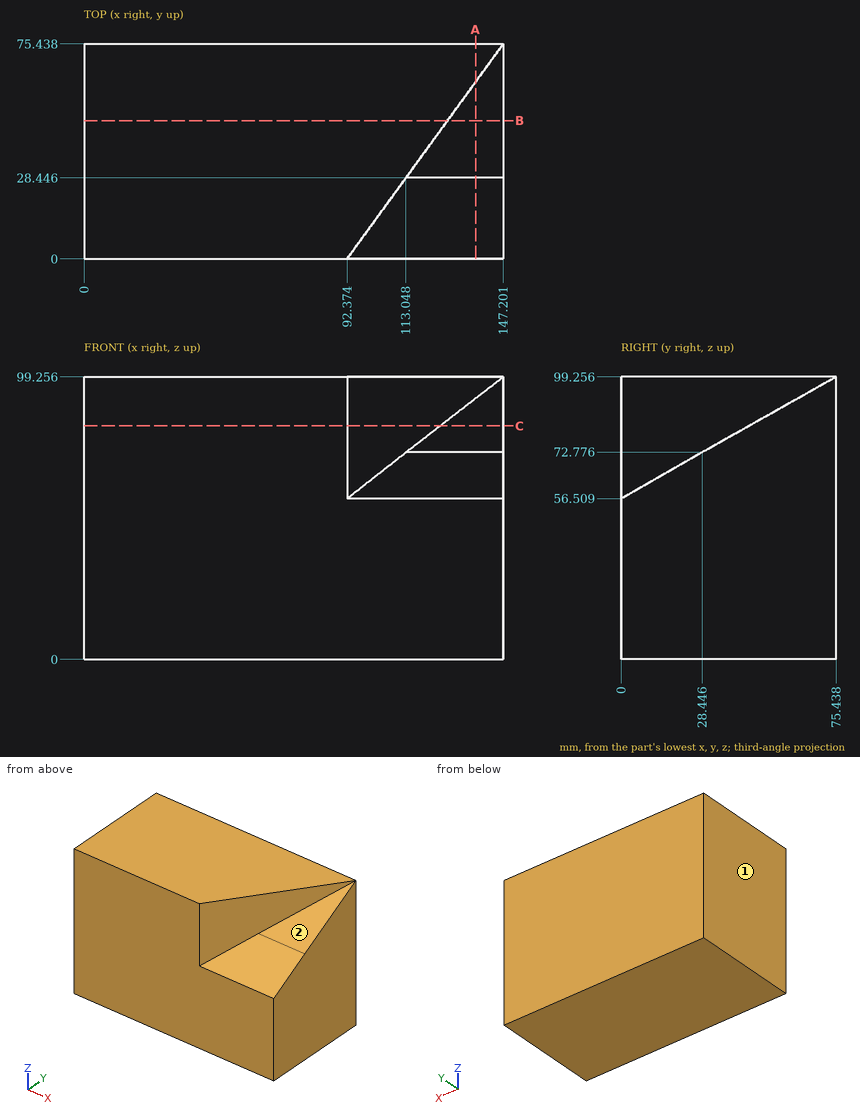
Source: three-view drawing plus pictorial views. Frame: mm from the lowest corner of the part. A direction names the side the tool comes from. Round coordinates to 2 decimals unless told otherwise and drop trailing zeros. Order: outer loops, then holes, each group sorted by start corner. A loop starts at its lowest first (then second) coordinate and runs counter-clockwise, first axis right, second up. Notation, with made-up numbers: (-1, 58) - (34, 58) arc R18 cw to (34, 76) - close; hole circle Ø7 at (87.25, -40). An arc over 180 degrees is marked (long way). Answer in a Markdown table with one row per item.
Item 1: Section query A-A (x = 137.5). Return the cut outline in (y, z) (1 decimal).
Model answer:
| item | result |
|---|---|
| outline | (0, 0) - (75.4, 0) - (75.4, 99.3) - (62.1, 99.3) - (62.1, 91.7) - (28.4, 72.8) - (0, 56.5) - close |
Item 2: Section query B-B (y = 48.5). Return the cut outline in (x, z) (1 decimal).
Model answer:
| item | result |
|---|---|
| outline | (0, 0) - (147.2, 0) - (147.2, 84.1) - (127.6, 84.1) - (127.6, 99.3) - (0, 99.3) - close |
Item 3: Reachability of the marked faces 1 and 2 from +Z, -Z, +X, -X, +Y, -Y: full face, straight path, thin tool, end or side. Return the list, or none.
Model answer:
| item | result |
|---|---|
| face 1 | +Z, -Z, -X, +Y, -Y |
| face 2 | +Z, +X, -Y |
Item 4: Pin query (flat end, axial travel): pin 1 (1.5 mm diameter, centred on x = 124, z = 62.5, fed in from -Y) (1 decimal); pin 2 (5 mm diameter, centred on x = 102, z = 75.5, fed in from -Y) (1 decimal). Return the tip coordinate at first contact, or that it passes through.
Model answer:
| item | result |
|---|---|
| pin 1 | stops at y = 9.2 |
| pin 2 | stops at y = 9.8 |
Item 5: Line query: line 1 (Y direction, x = 92.5, z = 59.5) (1 decimal); line 2 (X direction, y = 3, z = 77.5) (1 decimal); line 3 (Z direction, x = 135, y = 7). Output: solid intervals per line, ascending.
Model answer:
| item | result |
|---|---|
| line 1 | y = 0.2 to 75.4 |
| line 2 | x = 0 to 94.6 |
| line 3 | z = 0 to 60.51 |
Item 6: Section query C-C (z = 82). Return the cut outline in (x, y) (1 decimal), then the cut area to 3 significant figures.
Model answer:
| item | result |
|---|---|
| outline | (0, 0) - (92.4, 0) - (124.9, 44.8) - (147.2, 44.8) - (147.2, 75.4) - (0, 75.4) - close |
| area | 9,380 mm² |
